Input: part model. Units: mm. Frame: model coordinates. Face numbers are marked on the shaded views. A direction names the side the tool comes from. Coordinates: 2 decimals unless noted, no trailing zeros. Write each loop counter-clockwise with the first axis right and the second up, starting at its lowest first coordinate (ties: lowest second). Pieces come first, ordered by that corner, then holes.
1) Set-up query: the marked faces 4 and 5. Return all of +Z, -Z, +X, -X, +Y, -Y with unobstructed straight access to the full face (end or side cutting, diameter ignored); none if empty.
2) Section query A-A (x = -27.5). Output: boundary loops of the cut face in (y, z), then the cut area to 3 significant figures.
3) Section query B-B (y = 6). Output: boundary loops of the cut face in (x, z), then the cut area to 3 significant figures.
4) Section query D-D (y = -27.5). Output: boundary loops of the cut face in (x, z).
5) Pin query (flat end, axial travel): pin 1 Ø2.5 at (x, z) = (0, 114) entering from +Y; pin 2 Ø4 at (y, z) = (-24, 237) entering from -X; pin 3 Ø3.5 at (y, z) = (8.5, 148.5) entering from -X. Return the tip coordinate at first contact, or that it passes through.
6) Draft query along Y for the marked faces 1, 2 and 3. Return one class per face: pulls with the +Y half, pulls with the -Y half, needs draft (parallel to the pull), parting line crosses it, or undercut.
7) Line query: L1, parallel to Z at x = -1.5, y = -76.5; L2, parallel to X at y = -24.5, z = 21.5; L3, parallel to X at y = -41.5, z = 94. Output: solid intervals per line, ascending.
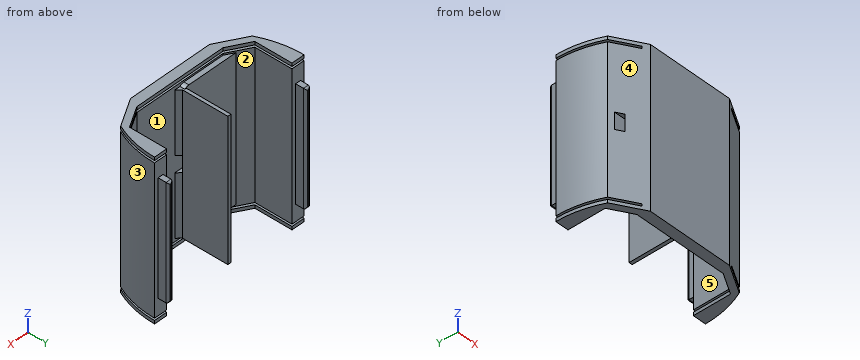
from build123d import *

# Parameters (mm, degrees)
BOSS_EXTRUDE1_DEPTH             = 240
CUT_EXTRUDE4_DEPTH              = 285.354710913
CUT_EXTRUDE4_DEPTH_BACK         = 285.354710913
CUT_EXTRUDE5_DEPTH              = 285.354710913
CUT_EXTRUDE5_DEPTH_BACK         = 285.354710913
SKETCH3_W                       = 3.3
SKETCH3_H                       = 170
BOSS_EXTRUDE4_REACH             = 286.355
SKETCH7_W                       = 213.4
SKETCH7_H                       = 5
BOSS_EXTRUDE4_DIRECTION_2_REACH = 286.355
CHAMFER7_SIZE                   = 6
SKETCH8_W                       = 5
SKETCH8_H                       = 213.4
BOSS_EXTRUDE5_DEPTH             = 120
CHAMFER8_SIZE                   = 6
CUT_EXTRUDE6_DEPTH              = 23
CUT_EXTRUDE6_DEPTH_BACK         = 176
SKETCH10_W                      = 25
SKETCH10_H                      = 6
BOSS_EXTRUDE6_DEPTH             = 90
FILLET1_R                       = 10
FILLET2_R                       = 10
SKETCH13_R                      = 1.2
CUT_EXTRUDE7_DEPTH              = 285.354710913
SKETCH14_R                      = 2
CUT_EXTRUDE8_DEPTH              = 47
CUT_EXTRUDE9_DEPTH              = 285.354710957
CUT_EXTRUDE9_DEPTH_BACK         = 285.354710957
SKETCH15_W                      = 272.433286574
SKETCH15_H                      = 99.158633553
SKETCH16_W                      = 8
SKETCH16_H                      = 173.4
BOSS_EXTRUDE7_DEPTH             = 15
FILLET3_R                       = 3


with BuildPart() as part:
    # Sketch1 → Boss-Extrude1 (new body)
    with BuildSketch(Plane.XY):
        with BuildLine():
            Line((-65, 90), (-108.301270189, 65))
            ThreePointArc((-108.301270189, 65), (-123.116211843, 0), (-108.301270189, -65))
            Line((-108.301270189, -65), (-65, -90))
            Line((-65, -90), (65, -90))
            Line((65, -90), (108.301270189, -65))
            ThreePointArc((108.301270189, -65), (123.116211843, 0), (108.301270189, 65))
            Line((108.301270189, 65), (65, 90))
            Line((65, 90), (-65, 90))
        make_face()
    extrude(amount=BOSS_EXTRUDE1_DEPTH)

    # Sketch2 → Cut-Extrude4 (cut, two sides: drawn at the far end of the back side and taken through both)
    with BuildSketch(Plane.XY.offset(240).offset(-CUT_EXTRUDE4_DEPTH_BACK)):
        Polygon((-70.980762114, 75), (70.980762114, 75), (103.116211843, 56.446589448), (103.116211843, -56.446589448), (70.980762114, -75), (-70.980762114, -75), (-103.116211843, -56.446589448), (-103.116211843, 56.446589448), align=None)
    extrude(amount=CUT_EXTRUDE4_DEPTH + CUT_EXTRUDE4_DEPTH_BACK, mode=Mode.SUBTRACT)

    # Sketch3 → Cut-Extrude5 (cut, two sides: drawn at the far end of the back side and taken through both)
    with BuildSketch(Plane(origin=(0, 0, 0), x_dir=(0, 0, -1), z_dir=(1, 0, 0)).offset(-CUT_EXTRUDE5_DEPTH_BACK)):
        with Locations((-233.35, 0)):
            Rectangle(SKETCH3_W, SKETCH3_H)
        with Locations((-6.65, 0)):
            Rectangle(SKETCH3_W, SKETCH3_H)
    extrude(amount=CUT_EXTRUDE5_DEPTH + CUT_EXTRUDE5_DEPTH_BACK, mode=Mode.SUBTRACT)

    # Boss-Extrude4: up to this face of the body (flat: up to its plane)
    boss_extrude4_end = Plane(part.part.faces().sort_by_distance((103.116211843, 0, 120))[0])
    # Sketch7 → Boss-Extrude4 (add, up to the picked face)
    with BuildSketch(Plane(origin=(0, 0, 0), x_dir=(0, 0, -1), z_dir=(1, 0, 0)), mode=Mode.PRIVATE) as boss_extrude4_sk1:
        with Locations((-120, 47.5)):
            Rectangle(SKETCH7_W, SKETCH7_H)
    boss_extrude4_tool1 = split(extrude(boss_extrude4_sk1.sketch, amount=BOSS_EXTRUDE4_REACH, mode=Mode.PRIVATE), bisect_by=boss_extrude4_end, keep=Keep.BOTH, mode=Mode.PRIVATE)
    add(boss_extrude4_tool1.solids().sort_by(Axis((0, 47.5, 120), (1, 0, 0)))[0])

    # Boss-Extrude4 direction 2: up to this face of the body (flat: up to its plane)
    boss_extrude4_direction_2_end = Plane(part.part.faces().sort_by_distance((-103.116211843, 0, 120))[0])
    # Sketch7 → Boss-Extrude4 direction 2 (add, up to the picked face)
    with BuildSketch(Plane(origin=(0, 0, 0), x_dir=(0, 0, -1), z_dir=(1, 0, 0)), mode=Mode.PRIVATE) as boss_extrude4_direction_2_sk1:
        with Locations((-120, 47.5)):
            Rectangle(SKETCH7_W, SKETCH7_H)
    boss_extrude4_direction_2_tool1 = split(extrude(boss_extrude4_direction_2_sk1.sketch, amount=-BOSS_EXTRUDE4_DIRECTION_2_REACH, mode=Mode.PRIVATE), bisect_by=boss_extrude4_direction_2_end, keep=Keep.BOTH, mode=Mode.PRIVATE)
    add(boss_extrude4_direction_2_tool1.solids().sort_by(Axis((0, 47.5, 120), (-1, 0, 0)))[0])

    # Chamfer7
    chamfer7_edges = [part.edges().sort_by_distance(p)[0] for p in [
        (-103.116211843, 45, 120),
        (103.116211843, 45, 120),
    ]]
    chamfer(chamfer7_edges, length=CHAMFER7_SIZE)

    # Sketch8 → Boss-Extrude5 (add)
    with BuildSketch(Plane(origin=(0, -75, 0), x_dir=(1, 0, 0), z_dir=(0, 1, 0))):
        with Locations((0, -120)):
            Rectangle(SKETCH8_W, SKETCH8_H)
    extrude(amount=BOSS_EXTRUDE5_DEPTH)

    # Chamfer8
    chamfer8_edges = [part.edges().sort_by_distance(p)[0] for p in [
        (2.5, -75, 120),
        (-2.5, -75, 120),
        (2.5, 45, 120),
        (-2.5, 45, 120),
    ]]
    chamfer(chamfer8_edges, length=CHAMFER8_SIZE)

    # Sketch10 → Cut-Extrude6 (cut, two sides: drawn at the far end of the back side and taken through both)
    with BuildSketch(Plane(origin=(0, 0, 0), x_dir=(0, 0, -1), z_dir=(1, 0, 0)).offset(-CUT_EXTRUDE6_DEPTH_BACK)):
        with Locations((-120, -72)):
            Rectangle(SKETCH10_W, SKETCH10_H)
    extrude(amount=CUT_EXTRUDE6_DEPTH + CUT_EXTRUDE6_DEPTH_BACK, mode=Mode.SUBTRACT)

    # Sketch12 → Boss-Extrude6 (add)
    with BuildSketch(Plane(origin=(0, 0, 0), x_dir=(0, 0, -1), z_dir=(1, 0, 0))):
        Polygon((-10.8, -67.5), (-229.2, -67.5), (-229.2, -75), (-132.5, -75), (-132.5, -69), (-107.5, -69), (-107.5, -75), (-10.8, -75), align=None)
    extrude(amount=-BOSS_EXTRUDE6_DEPTH)

    # Fillet1
    # the kernel refuses this fillet: 10 mm, written as the material it takes off along each edge
    with BuildSketch(Plane(origin=(0, -75, 10.8), x_dir=(-1, 0, 0), z_dir=(0, 1, 0))) as fillet1_piece_1:
        with BuildLine():
            CenterArc((6.614378278, 10), FILLET1_R, 228.590377891, 41.409622109)
            Line((0, 2.5), (-0.132287566, 2.35))
            ThreePointArc((-0.132287566, 2.35), (-0.2, 1.25), (-0.2, 0))
            Line((-0.2, 0), (0, -0.2))
            Line((0, -0.2), (6.614378278, -0.2))
            Line((6.614378278, -0.2), (6.614378278, 0))
        make_face()
    extrude(amount=24.035945694, mode=Mode.SUBTRACT)

    # Fillet2
    # the kernel refuses this fillet: 10 mm, written as the material it takes off along each edge
    with BuildSketch(Plane(origin=(0, -50.964054306, 229.2), x_dir=(0, 0, -1), z_dir=(0, -1, 0))) as fillet2_piece_1:
        with BuildLine():
            CenterArc((10, -6.614378278), FILLET2_R, 138.590377891, 41.409622109)
            Line((0, -6.614378278), (-0.2, -6.614378278))
            Line((-0.2, -6.614378278), (-0.2, 0))
            Line((-0.2, 0), (0, 0.2))
            ThreePointArc((0, 0.2), (1.25, 0.2), (2.35, 0.132287566))
            Line((2.35, 0.132287566), (2.5, 0))
        make_face()
    extrude(amount=24.035945694, mode=Mode.SUBTRACT)

    # Sketch13 → Cut-Extrude7 (cut, through all)
    with BuildSketch(Plane(origin=(0, 0, 0), x_dir=(0, 0, -1), z_dir=(1, 0, 0))):
        with Locations((-173.35, 62.5)):
            Circle(SKETCH13_R)
        with Locations((-66.65, 62.5)):
            Circle(SKETCH13_R)
    extrude(amount=-CUT_EXTRUDE7_DEPTH, mode=Mode.SUBTRACT)

    # Sketch14 → Cut-Extrude8 (cut)
    with BuildSketch(Plane(origin=(0, 50, 0), x_dir=(1, 0, 0), z_dir=(0, 1, 0))):
        with Locations(Location((-41.18, -120, 0), (0, 0, 270))):
            Circle(SKETCH14_R)
    extrude(amount=-CUT_EXTRUDE8_DEPTH, mode=Mode.SUBTRACT)

    # Sketch15 → Cut-Extrude9 (cut, two sides: drawn at the far end of the back side and taken through both)
    with BuildSketch(Plane.XY.offset(-CUT_EXTRUDE9_DEPTH_BACK)):
        with Locations((1.391256338, 49.579316777)):
            Rectangle(SKETCH15_W, SKETCH15_H)
    extrude(amount=CUT_EXTRUDE9_DEPTH + CUT_EXTRUDE9_DEPTH_BACK, mode=Mode.SUBTRACT)

    # Sketch16 → Boss-Extrude7 (add)
    with BuildSketch(Plane(origin=(0, 0, 0), x_dir=(1, 0, 0), z_dir=(0, 1, 0))):
        with Locations((-113.116211843, -120)):
            Rectangle(SKETCH16_W, SKETCH16_H)
        with Locations((113.116211843, -120)):
            Rectangle(SKETCH16_W, SKETCH16_H)
    extrude(amount=BOSS_EXTRUDE7_DEPTH)

    # Fillet3
    fillet3_edges = [part.edges().sort_by_distance(p)[0] for p in [
        (-117.116211843, 15, 120),
        (-113.116211843, 15, 206.7),
        (-109.116211843, 15, 120),
        (-113.116211843, 15, 33.3),
        (109.116211843, 15, 120),
        (113.116211843, 15, 206.7),
        (117.116211843, 15, 120),
        (113.116211843, 15, 33.3),
    ]]
    fillet(fillet3_edges, radius=FILLET3_R)


solid = part.part
Answer:
1. face 4: +Z, -Z, -X, -Y
1. face 5: +Z, -Z, +Y
2. outline: (-90, 0) - (-75, 0) - (-75, 5) - (-85, 5) - (-85, 8.3) - (-75, 8.3) - (-75, 10.8) - (-67.5, 10.8) - (-67.5, 229.2) - (-75, 229.2) - (-75, 231.7) - (-85, 231.7) - (-85, 235) - (-75, 235) - (-75, 240) - (-90, 240) - close; hole (-75, 107.5) - (-69, 107.5) - (-69, 132.5) - (-75, 132.5) - close
2. area: 5,020 mm2
3. outline: (-117.12, 33.3) - (-109.12, 33.3) - (-109.12, 206.7) - (-117.12, 206.7) - close; (109.12, 33.3) - (117.12, 33.3) - (117.12, 206.7) - (109.12, 206.7) - close
3. area: 2,770 mm2
4. outline: (-120.57, 0) - (-103.12, 0) - (-103.12, 5) - (-120.57, 5) - close; (-120.57, 8.3) - (-103.12, 8.3) - (-103.12, 231.7) - (-120.57, 231.7) - close; (-120.57, 235) - (-103.12, 235) - (-103.12, 240) - (-120.57, 240) - close; (-2.5, 13.3) - (2.5, 13.3) - (2.5, 226.7) - (-2.5, 226.7) - close; (103.12, 0) - (120.57, 0) - (120.57, 5) - (103.12, 5) - close; (103.12, 8.3) - (120.57, 8.3) - (120.57, 231.7) - (103.12, 231.7) - close; (103.12, 235) - (120.57, 235) - (120.57, 240) - (103.12, 240) - close
5. pin 1: stops at y = 0
5. pin 2: stops at x = -121.49
5. pin 3: stops at x = -117.12
6. face 1: undercut
6. face 2: pulls with the +Y half
6. face 3: pulls with the -Y half
7. L1: z = 0 to 5, 8.3 to 231.7, 235 to 240
7. L2: x = -121.1 to -103.12, -2.5 to 2.5, 103.12 to 121.1
7. L3: x = -117.26 to -103.12, -2.5 to 2.5, 103.12 to 117.26
